Design review of the part shown in the three views and the two pictorial views. Dimensions are in mm from the part's minimum x, y and z. A direction names the side the tool comes from. Round coordinates to 2 decimals unless told otherwise and drop trailing zeros. Loops run counter-clockwise (first coordinate to the right, second up) from the corner with the lowest first, then second, coordinate; pieces in that order, holes last.
1. Clearance check with flat-ended pins moving along their axes: pin 1 Ø5 at (y, z) = (47, 8) entering from +X; pin 2 Ø2 at (x, z) = (24.5, 16) entering from +Y; pin 3 Ø12 at (x, y) = (6.5, 53) entering from -Z; pin 4 Ø5 at (y, z) = (40, 11.5) entering from -X. State where each tip first meets the part, or that it passes through.
2. To check wall thickness, follow line 1 along Y through (x, z) = (30, 11.75); line 2 along X through (y, z) = (30.5, 14.5); line 3 along Z through (x, y) = (33, 37). State the ranges of each line that lie inside material, in increasing order.
3. Consider section A-A on z = 14.5. State the section outline as (x, y) points.
4. Tool access review of the marked faces 4 and 5: name each direction out of +Z, -Z, +X, -X, +Y, -Y from which nothing blocks a thin tool from reaching the whole face with its end or side.
5. Draft analysis for pull direction Y (two halves, no side actions). For the marked faces 1, 2 and 3, state which applies: released by +Y, released by -Y, zero draft, split by the parting line, or undercut.
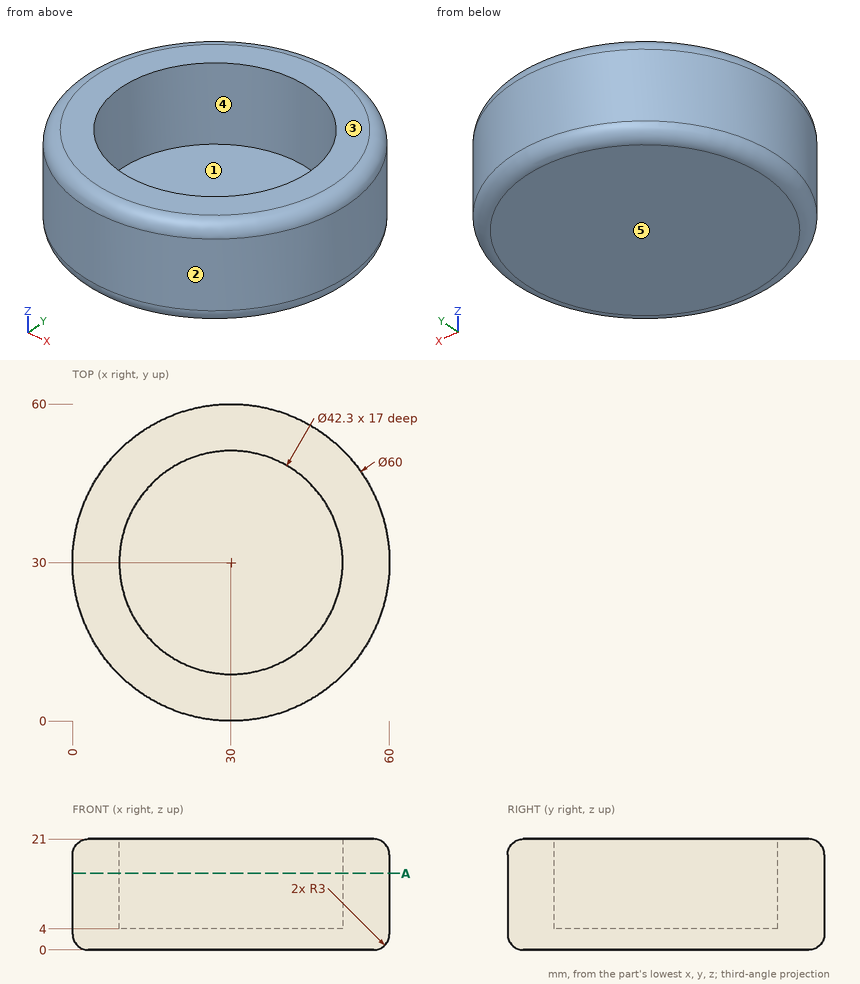
Resolved:
1. pin 1: stops at x = 56.26
1. pin 2: stops at y = 59.66
1. pin 3: stops at z = 0
1. pin 4: stops at x = 0.95
2. line 1: y = 0 to 8.85, 51.15 to 60
2. line 2: x = 0 to 8.86, 51.14 to 60
2. line 3: z = 0 to 4
3. outline: circle Ø60 at (30, 30); hole circle Ø42.3 at (30, 30)
4. face 4: +Z
4. face 5: -Z, +X, -X, +Y, -Y
5. face 1: undercut
5. face 2: split by the parting line
5. face 3: zero draft
